```python
from build123d import *

# Parameters (mm, degrees)
F0_W     = 114
F0_H     = 72
F0_W_2   = 110
F0_H_2   = 68
F0_W_3   = 1
F1_DEPTH = 1.6
F2_DEPTH = 3
F3_W     = 114
F3_H     = 72
F3_W_2   = 111
F3_H_2   = 69
F4_DEPTH = 1.5
F5_DEPTH = 3
F3_W_3   = 1
F6_DEPTH = 3


with BuildPart() as f1:
    # F0 (on Top) → F1 (new body)
    with BuildSketch(Plane.XY):
        with BuildLine():
            Line((58, 39), (-58, 39))
            ThreePointArc((-58, 39), (-59.4142135624, 38.4142135624), (-60, 37))
            Line((-60, 37), (-60, -37))
            ThreePointArc((-60, -37), (-59.4142135624, -38.4142135624), (-58, -39))
            Line((-58, -39), (58, -39))
            ThreePointArc((58, -39), (59.4142135624, -38.4142135624), (60, -37))
            Line((60, -37), (60, 37))
            ThreePointArc((60, 37), (59.4142135624, 38.4142135624), (58, 39))
        make_face()
        Polygon((58, 37), (58, 36), (58, -36), (58, -37), (-58, -37), (-58, 37), align=None, mode=Mode.SUBTRACT)
        Polygon((-57, -36), (-57, 36), (57, 36), (58, 36), (58, 37), (-58, 37), (-58, -37), (58, -37), (58, -36), (57, -36), align=None)
        Rectangle(F0_W, F0_H)
        Rectangle(F0_W_2, F0_H_2, mode=Mode.SUBTRACT)
        with Locations((57.5, 0)):
            Rectangle(F0_W_3, F0_H)
    extrude(amount=F1_DEPTH)

    # F0 (on Top) → F2 (join)
    with BuildSketch(Plane.XY):
        Polygon((-57, -36), (-57, 36), (57, 36), (58, 36), (58, 37), (-58, 37), (-58, -37), (58, -37), (58, -36), (57, -36), align=None)
    extrude(amount=-F2_DEPTH)

    # F3 (on face) → F4 (join)
    with BuildSketch(Plane(origin=(0, 0, -3), x_dir=(1, 0, 0), z_dir=(0, 0, -1))):
        Rectangle(F3_W, F3_H)
        Rectangle(F3_W_2, F3_H_2, mode=Mode.SUBTRACT)
    extrude(amount=F4_DEPTH)

    # F5 (add): a face of the model
    f5_faces = [f1.faces().sort_by_distance(p)[0] for p in [
        (-57.1375936045, 0, -3),
    ]]
    extrude(f5_faces, amount=F5_DEPTH)

    # F3 (on face) → F6 (join)
    with BuildSketch(Plane(origin=(0, 0, -3), x_dir=(1, 0, 0), z_dir=(0, 0, -1))):
        with Locations((57.5, 0)):
            Rectangle(F3_W_3, F3_H)
    extrude(amount=F6_DEPTH)


solid = f1.part
```
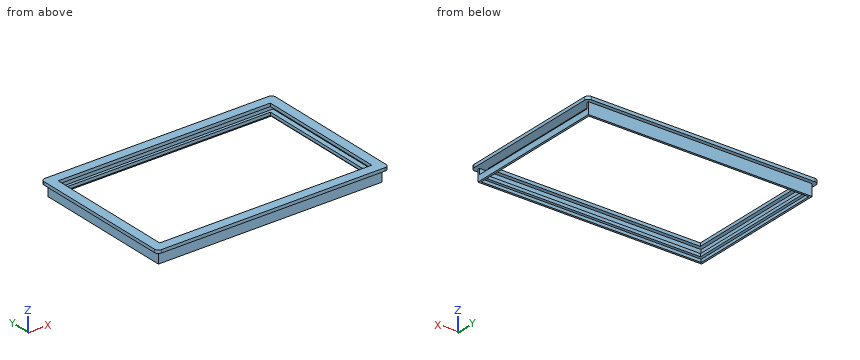
Model file for the job. Use its own axes, mm. Give positions to 0.01 mm unless a question says otherwise; leave off trailing zeros. Order: outer loops, then holes, each group sorted by start corner. A loop starts at its lowest first (then second) coordinate and runs counter-clockwise, first axis right, second up.
1) Saw through at B-B, the plane x = -51. Write the cut outline in (y, z).
2) Saw through at C-C, the plane z = -1.5. Write the cut outline in (x, y).
3) Pin check, flat tips, straight feed: pin 1 (1.8 mm diameter, centred on y = 13.5, z = -4, fed in from -X); pin 2 (23.5 mm diameter, centred on x = -6, y = 11, fed in from -Z); pin 3 (1 mm diameter, centred on y = -22.5, z = -3, fed in from +X); pin 4 (3 mm diameter, centred on x = -4, z = -2, fed in from -Y). Stop position of each tip, or through.
4) Wall check: probe 1 along Y at (x, z) = (16, -1.5); probe 2 along X at (y, z) = (-27, 0.5); probe 3 along Y at (x, z) = (-25, 0.5). Give the ranges that are in metal, low to high.
5) Saw through at A-A, the plane y = -12. Write the cut outline in (x, z), then the cut area to 3 significant figures.
Computed:
1. outline: (-39, 0) - (-37, 0) - (-37, -6) - (-36, -6) - (-36, -4.5) - (-34.5, -4.5) - (-34.5, -3) - (-36, -3) - (-36, 0) - (-34, 0) - (-34, 1.6) - (-39, 1.6) - close; (34, 0) - (36, 0) - (36, -3) - (34.5, -3) - (34.5, -4.5) - (36, -4.5) - (36, -6) - (37, -6) - (37, 0) - (39, 0) - (39, 1.6) - (34, 1.6) - close
2. outline: (-58, -37) - (58, -37) - (58, -36) - (-57, -36) - (-57, 36) - (58, 36) - (58, 37) - (-58, 37) - close
3. pin 1: stops at x = -58
3. pin 2: passes through
3. pin 3: stops at x = 58
3. pin 4: stops at y = -37
4. probe 1: y = -37 to -36, 36 to 37
4. probe 2: x = -60 to -55, 55 to 60
4. probe 3: y = -39 to -34, 34 to 39
5. outline: (-60, 0) - (-58, 0) - (-58, -6) - (-57, -6) - (-57, -4.5) - (-55.5, -4.5) - (-55.5, -3) - (-57, -3) - (-57, 0) - (-55, 0) - (-55, 1.6) - (-60, 1.6) - close; (55, 0) - (60, 0) - (60, 1.6) - (55, 1.6) - close; (55.5, -4.5) - (57, -4.5) - (57, -6) - (58, -6) - (58, -3) - (55.5, -3) - close
5. area: 29.5 mm2
